Answer from the drawing. Dimensions are ordinates in mm from the lowest x, y and z of the part. A direction names the side the tool comes from. Give positions to 0.01 mm unless a question says otherwise; leave off trailing zeros. Order: outer loops, then holes, each group sorted by start corner. A loop starts at its lowest first (then second) coordinate and runs counter-clockwise, first axis right, second up.
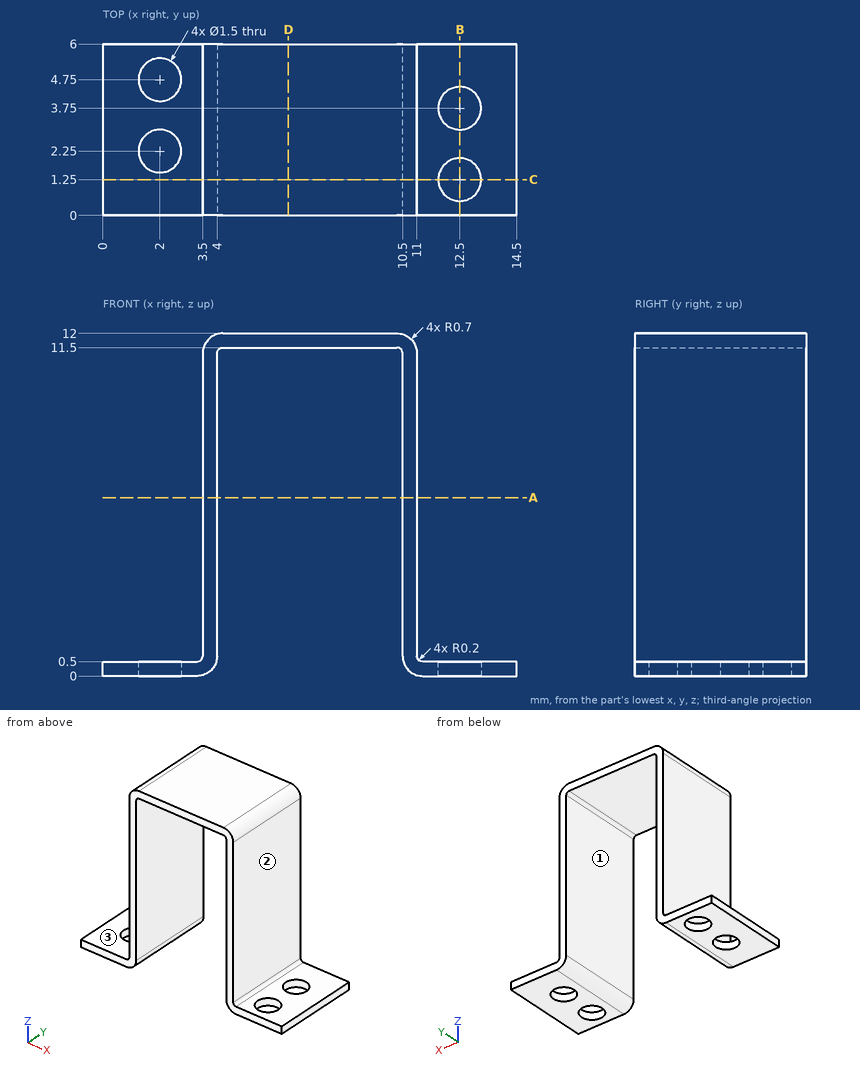
1. The part is cut by section D-D (x = 6.5). Write down the section's boundary in (y, z), then the cut area to 3 significant figures.
Findings below:
outline: (0, 11.5) - (6, 11.5) - (6, 12) - (0, 12) - close
area: 3.00 mm2
2. Given P1, Ø0.9, axis at x = 12.5, y = 1.25, coming from the +Z side; P2, Ø1.5, axis at y = 5, z = 5, coming from the +X side; P3, Ø2.5, axis at x = 12.5, y = 3.75, coming from the +Z side; P4, Ø3, axis at x = 2.5, y = 2, coming from the +Z side, each flat-ended and moving along its own axis, determine where each tip first touches the part or whether it passes through.
Findings below:
P1: passes through
P2: stops at x = 11
P3: stops at z = 0.5
P4: stops at z = 11.97
3. Which of the six approach directions +Z, -Z, +X, -X, +Y, -Y give full straight-line access (tool end or side, diameter ignored) to the marked faces 1, 2 and 3?
Findings below:
face 1: -Z, +Y, -Y
face 2: +Z, +X, +Y, -Y
face 3: +Z, -X, +Y, -Y
4. The part is cut by section B-B (x = 12.5). Write down the section's boundary in (y, z).
Findings below:
outline: (0, 0) - (0.5, 0) - (0.5, 0.5) - (0, 0.5) - close; (2, 0) - (3, 0) - (3, 0.5) - (2, 0.5) - close; (4.5, 0) - (6, 0) - (6, 0.5) - (4.5, 0.5) - close
5. The part is cut by section C-C (y = 1.25). Write down the section's boundary in (x, z), then the cut area to 3 significant figures.
Findings below:
outline: (0, 0) - (3.3, 0) arc R0.7 ccw to (4, 0.7) - (4, 11.3) arc R0.2 cw to (4.2, 11.5) - (10.3, 11.5) arc R0.2 cw to (10.5, 11.3) - (10.5, 0.7) arc R0.7 ccw to (11.2, 0) - (11.75, 0) - (11.75, 0.5) - (11.2, 0.5) arc R0.2 cw to (11, 0.7) - (11, 11.3) arc R0.7 ccw to (10.3, 12) - (4.2, 12) arc R0.7 ccw to (3.5, 11.3) - (3.5, 0.7) arc R0.2 cw to (3.3, 0.5) - (0, 0.5) - close; (13.25, 0) - (14.5, 0) - (14.5, 0.5) - (13.25, 0.5) - close
area: 17.6 mm2
6. The part is cut by section A-A (z = 6.25). Write down the section's boundary in (x, y).
Findings below:
outline: (3.5, 0) - (4, 0) - (4, 6) - (3.5, 6) - close; (10.5, 0) - (11, 0) - (11, 6) - (10.5, 6) - close
7. Straight lines are drawn through the part: probe 1 along Y at (x, z) = (12.5, 0.35); probe 2 along Y at (x, z) = (2, 0.25); probe 3 along X at (y, z) = (2.6, 7.75). For each, find the intervals that lie inside material, in ascending order.
Findings below:
probe 1: y = 0 to 0.5, 2 to 3, 4.5 to 6
probe 2: y = 0 to 1.5, 3 to 4, 5.5 to 6
probe 3: x = 3.5 to 4, 10.5 to 11
